from build123d import *

# Parameters (mm, degrees)
ESBO_O1_W                = 40
ESBO_O1_H                = 50
RESSALTO_EXTRUS_O1_DEPTH = 2
ESBO_O2_W                = 40
ESBO_O2_H                = 20
ESBO_O2_H_2              = 15
RESSALTO_EXTRUS_O2_DEPTH = 15
ESBO_O3_R                = 12.5
CORTE_EXTRUS_O1_DEPTH    = 22
ESBO_O4_R                = 11
CORTE_EXTRUS_O2_DEPTH    = 22
CORTE_EXTRUS_O3_DEPTH    = 22
ESBO_O6_W                = 5
ESBO_O6_H                = 2
CORTE_EXTRUS_O4_DEPTH    = 51.139804547
FILETE1_R                = 2
FILETE2_R                = 2
FILETE3_R                = 2
FILETE4_R                = 2
FILETE5_R                = 2
FILETE6_R                = 2
FILETE7_R                = 2
FILETE8_R                = 2


with BuildPart() as part:
    # Esboço1 → Ressalto-extrusão1 (new body)
    with BuildSketch(Plane(origin=(0, 0, 0), x_dir=(1, 0, 0), z_dir=(0, 1, 0))):
        Rectangle(ESBO_O1_W, ESBO_O1_H)
    extrude(amount=RESSALTO_EXTRUS_O1_DEPTH)

    # Esboço2 → Ressalto-extrusão2 (add)
    with BuildSketch(Plane(origin=(0, 2, 0), x_dir=(1, 0, 0), z_dir=(0, 1, 0))):
        with Locations((0, 15)):
            Rectangle(ESBO_O2_W, ESBO_O2_H)
        with Locations((0, -17.5)):
            Rectangle(ESBO_O2_W, ESBO_O2_H_2)
    extrude(amount=RESSALTO_EXTRUS_O2_DEPTH)

    # Esboço3 → Corte-extrusão1 (cut)
    with BuildSketch(Plane.XY.offset(25)):
        with Locations((0, 17)):
            Circle(ESBO_O3_R)
    extrude(amount=-CORTE_EXTRUS_O1_DEPTH, mode=Mode.SUBTRACT)

    # Esboço4 → Corte-extrusão2 (cut)
    with BuildSketch(Plane(origin=(0, 0, -25), x_dir=(-1, 0, 0), z_dir=(0, 0, -1))):
        with Locations((0, 17)):
            Circle(ESBO_O4_R)
    extrude(amount=-CORTE_EXTRUS_O2_DEPTH, mode=Mode.SUBTRACT)

    # Esboço5 → Corte-extrusão3 (cut)
    with BuildSketch(Plane(origin=(0, 2, 0), x_dir=(1, 0, 0), z_dir=(0, 1, 0))):
        with BuildLine():
            Line((-12.449166755, 1.40771236), (12.633097958, 1.40771236))
            ThreePointArc((12.633097958, 1.40771236), (16.682554855, -2.641744537), (12.633097958, -6.691201435))
            Line((12.633097958, -6.691201435), (-12.449166755, -6.691201435))
            ThreePointArc((-12.449166755, -6.691201435), (-16.498623653, -2.641744537), (-12.449166755, 1.40771236))
        make_face()
    extrude(amount=-CORTE_EXTRUS_O3_DEPTH, mode=Mode.SUBTRACT)

    # Esboço6 → Corte-extrusão4 (cut, through all)
    with BuildSketch(Plane.ZY.offset(20)):
        with Locations((-15, 3)):
            Rectangle(ESBO_O6_W, ESBO_O6_H)
        with Locations((17.5, 3)):
            Rectangle(ESBO_O6_W, ESBO_O6_H)
    extrude(amount=-CORTE_EXTRUS_O4_DEPTH, mode=Mode.SUBTRACT)

    # Filete1
    filete1_edges = [part.edges().sort_by_distance(p)[0] for p in [
        (-20, 9.5, 10),
    ]]
    fillet(filete1_edges, radius=FILETE1_R)

    # Filete2
    filete2_edges = [part.edges().sort_by_distance(p)[0] for p in [
        (-20, 9.5, -5),
    ]]
    fillet(filete2_edges, radius=FILETE2_R)

    # Filete3
    filete3_edges = [part.edges().sort_by_distance(p)[0] for p in [
        (-20, 8.5, 25),
    ]]
    fillet(filete3_edges, radius=FILETE3_R)

    # Filete4
    filete4_edges = [part.edges().sort_by_distance(p)[0] for p in [
        (-20, 8.5, -25),
    ]]
    fillet(filete4_edges, radius=FILETE4_R)

    # Filete5
    filete5_edges = [part.edges().sort_by_distance(p)[0] for p in [
        (20, 8.5, -25),
    ]]
    fillet(filete5_edges, radius=FILETE5_R)

    # Filete6
    filete6_edges = [part.edges().sort_by_distance(p)[0] for p in [
        (20, 9.5, 10),
    ]]
    fillet(filete6_edges, radius=FILETE6_R)

    # Filete7
    filete7_edges = [part.edges().sort_by_distance(p)[0] for p in [
        (20, 9.5, -5),
    ]]
    fillet(filete7_edges, radius=FILETE7_R)

    # Filete8
    filete8_edges = [part.edges().sort_by_distance(p)[0] for p in [
        (20, 8.5, 25),
    ]]
    fillet(filete8_edges, radius=FILETE8_R)


solid = part.part
For this review, take the finished solid that the model builds, in its own axes (mm). A direction names the side the tool comes from. Give positions to 0.01 mm unless a question says otherwise; leave off trailing zeros. Loops run counter-clockwise (first coordinate to the right, second up) from the corner with the lowest first, then second, coordinate; pieces in that order, holes last.
Item 1: Take a section at A-A, the plane x = 0. State the section outline as (y, z) points, and give its area (3 significant figures).
Item 2: For line 1 along Z through (x, y) = (10.5, 3.5); line 2 along Z through (x, y) = (17, 9.75); line 3 along Z through (x, y) = (-12, 1), list the stretches that pass through material, from the lowest coordinate up.
Item 3: Take a section at C-C, the plane y = 9.5. State the section outline as (x, z) points.
Item 4: Take a section at D-D, the plane z = 3. State the section outline as (x, y) points, and give its area (3 significant figures).
Item 5: Take a section at B-B, the plane y = 1. State the section outline as (x, z) points, and give its area (3 significant figures).
Item 6: Draft analysis for pull direction Y (two halves, no side actions). For faces 1 (the flat face through (-16, 17, -15)), 2 (the flat face through (0, 3, 15)), 3 (the cylindrical face through (-19.43, 9.6, -5.6)), state which applies: +Y half, -Y half, draft (parallel to the pull), parting line (faces both ways), or undercut.
Item 7: Tool access review of faces 4 (the flat face through (0, 1, -1.408)), 5 (the flat face through (0, 2, 17)), 6 (the flat face through (0, 4, -5)): name each direction out of +Z, -Z, +X, -X, +Y, -Y from which nothing blocks a thin tool from reaching the whole face with its end or side.
Item 8: Insertion check: pin 1 (2.5 mm diameter, centred on x = -6.5, z = 17, fed in from +Y); pin 2 (4 mm diameter, centred on x = 2.5, z = 18.5, fed in from +Y); pin 3 (2.5 mm diameter, centred on x = -2.5, z = -15, fed in from +Y). Each pin has a flat end and moves straight along its axis. Give the tip position at first contact, or say it passes through.
Calculated:
1. outline: (0, -25) - (6, -25) - (6, -5) - (2, -5) - (2, -1.41) - (0, -1.41) - close; (0, 6.69) - (2, 6.69) - (2, 10) - (4.5, 10) - (4.5, 25) - (0, 25) - close; hole (2, -17.5) - (4, -17.5) - (4, -12.5) - (2, -12.5) - close; hole (2, 15) - (4, 15) - (4, 20) - (2, 20) - close
1. area: 181 mm2
2. line 1: z = -25 to -17.5, -12.5 to -5, 10 to 15, 20 to 25
2. line 2: z = -25 to -5, 10 to 25
2. line 3: z = -25 to -1.41, 6.69 to 25
3. outline: (-20, -23) arc R2 ccw to (-18, -25) - (-8.05, -25) - (-8.05, -5) - (-18, -5) arc R2 ccw to (-20, -7) - close; (-20, 12) arc R2 ccw to (-18, 10) - (-10, 10) - (-10, 25) - (-18, 25) arc R2 ccw to (-20, 23) - close; (8.05, -25) - (18, -25) arc R2 ccw to (20, -23) - (20, -7) arc R2 ccw to (18, -5) - (8.05, -5) - close; (10, 10) - (18, 10) arc R2 ccw to (20, 12) - (20, 23) arc R2 ccw to (18, 25) - (10, 25) - close
4. outline: (-20, 0) - (-16.48, 0) - (-16.48, 2) - (-20, 2) - close; (16.67, 0) - (20, 0) - (20, 2) - (16.67, 2) - close
4. area: 13.7 mm2
5. outline: (-20, -23) arc R2 ccw to (-18, -25) - (18, -25) arc R2 ccw to (20, -23) - (20, 23) arc R2 ccw to (18, 25) - (-18, 25) arc R2 ccw to (-20, 23) - close; hole (-12.45, -1.41) - (12.63, -1.41) arc R4.05 ccw to (12.63, 6.69) - (-12.45, 6.69) arc R4.05 ccw to start
5. area: 1,740 mm2
6. face 1: +Y half
6. face 2: undercut
6. face 3: draft
7. face 4: +Y, -Y
7. face 5: +X, -X
7. face 6: +X, -X, +Y
8. pin 1: stops at y = 7.19
8. pin 2: stops at y = 5.34
8. pin 3: stops at y = 6.66
